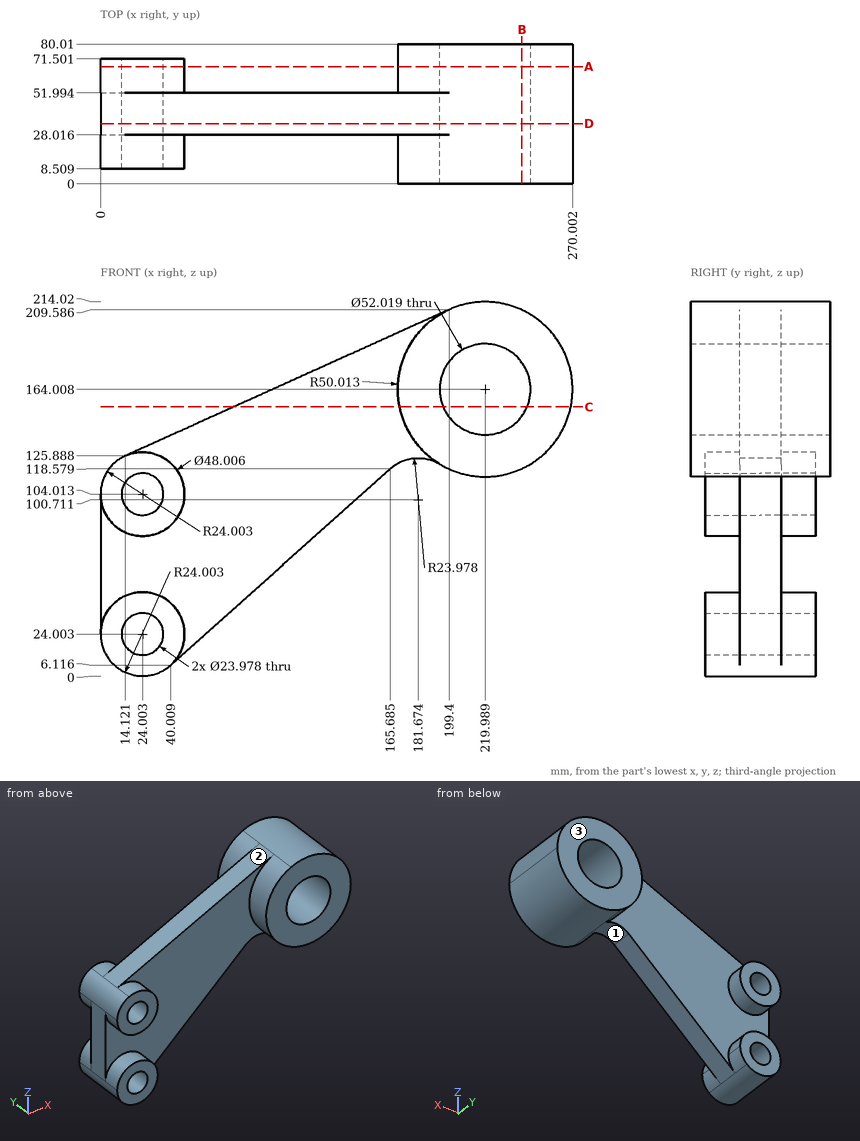
Print and shaded views of the part. All mm, measured from the part's lowest x, y and z. Give positions to 0.01 mm unless a question says otherwise; leave off trailing zeros. Write each loop counter-clockwise with the first axis right and the second up, starting at its lowest first coordinate (ties: lowest second). Pieces come first, ordered by that corner, then holes. Notation, with made-up numbers: (24, 54) - (82, 54) arc R22 cw to (82, 86) - close; hole circle Ø2 at (57.5, 20.5). An arc over 180 degrees is marked (long way). Put each result on its own line as item: value.
(1) Drop flat-ended pins along their axis: pin 1 Ø6 at (y, z) = (51, 73.5) entering from +X; pin 2 Ø10 at (x, z) = (94.5, 169.5) entering from -Y; pin 3 Ø12 at (y, z) = (52.5, 97.5) entering from +X; pin 4 Ø2 at (x, z) = (80.5, 148) entering from +Y. Give the stop position or say it passes through.
Working result:
pin 1: x = 118.66
pin 2: through
pin 3: x = 148.81
pin 4: y = 51.99
(2) Pull direction X, two halves, no side cores. Call the marked faces 1, 2 and 3: released by +X, released by -X, zero draft, split by the parting line, or undercut.
Working result:
face 1: undercut
face 2: released by -X
face 3: zero draft
(3) Saw through at C-C (z = 154). List the corners of the cut face in (x, y), then the cut area to 3 significant figures.
Working result:
outline: (76.35, 28.02) - (170.99, 28.02) - (170.99, 0) - (195.98, 0) - (195.98, 80.01) - (170.99, 80.01) - (170.99, 51.99) - (76.35, 51.99) - close; (244, 0) - (268.99, 0) - (268.99, 80.01) - (244, 80.01) - close
area: 6,270 mm^2
(4) Saw through at A-A (y = 67). List the corners of the cut face in (x, z) (1 decimal), then the cut area to 3 significant figures.
Working result:
outline: circle Ø48 at (24, 104); (40, 6.1) arc R24 ccw to (48, 24) arc R24 ccw (long way) to start; circle Ø100 at (220, 164); hole circle Ø24 at (24, 24); hole circle Ø24 at (24, 104); hole circle Ø52 at (220, 164)
area: 8,450 mm^2
(5) Saw through at D-D (y = 34.5). List the corners of the cut face in (x, z) (1 decimal), then the cut area to 3 significant figures.
Working result:
outline: (0, 24) arc R24 ccw to (40, 6.1) - (165.7, 118.6) arc R24 cw to (194.1, 121.2) arc R50 ccw (long way) to (199.4, 209.6) - (14.1, 125.9) arc R24 ccw to (0, 104) - close; hole circle Ø24 at (24, 24); hole circle Ø24 at (24, 104); hole circle Ø52 at (220, 164)
area: 23,500 mm^2
(6) Saw through at B-B (x = 241). List the corners of the cut face in (y, z).
Working result:
outline: (0, 118.62) - (80.01, 118.62) - (80.01, 148.68) - (0, 148.68) - close; (0, 179.34) - (80.01, 179.34) - (80.01, 209.39) - (0, 209.39) - close
(7) Wall check: L1, parallel to Z at x = 27, y = 10 (1 decimal); L2, parallel to Z at x = 24.5, y = 47.5 (1 decimal); L3, parallel to Z at x = 42.5, y = 64 (1 decimal). Give the ranges that are in metal, low to high.
Working result:
L1: 0.2 to 12.4, 35.6 to 47.8, 80.2 to 92.4, 115.6 to 127.8
L2: 0 to 12, 36 to 92, 116 to 130.6
L3: 8.7 to 39.3, 88.7 to 119.3
